```python
from build123d import *

# Parameters (mm, degrees)
SKETCH_1_W           = 40
SKETCH_1_H           = 15
EXTRUDE_1_DEPTH      = 5
CUT_EXTRUDE_START    = 5
SKETCH_2_R           = 5
SKETCH_2_R_2         = 1.5
CUT_EXTRUDE_1_DEPTH  = 5
EXTRUDE_3_DEPTH      = 8.75
EXTRUDE_3_DEPTH_BACK = 3.75
SKETCH_6_W           = 12.5
SKETCH_6_H           = 4
EXTRUDE_START        = 7.5
EXTRUDE_4_DEPTH      = 4
EXTRUDE_START_2      = -7.5
EXTRUDE_5_DEPTH      = 4
CUT_EXTRUDE_START_2  = 7.5
SKETCH_10_R          = 2.75
CUT_EXTRUDE_3_DEPTH  = 15
CUT_EXTRUDE_START_3  = -3.5
CUT_EXTRUDE_4_DEPTH  = 7
CHAMFER_1_SIZE       = 1


with BuildPart() as part:
    # 草图1 → 凸台-拉伸1 (new body)
    with BuildSketch(Plane(origin=(0, 0, 0), x_dir=(1, 0, 0), z_dir=(0, 1, 0))):
        Rectangle(SKETCH_1_W, SKETCH_1_H)
    extrude(amount=EXTRUDE_1_DEPTH)

    # 草图2 → 切除-拉伸1 (cut)
    with BuildSketch(Plane(origin=(0, 0, 0), x_dir=(1, 0, 0), z_dir=(0, 1, 0)).offset(CUT_EXTRUDE_START)):
        with Locations(Location((0, 0, 0), (0, 0, 90))):
            Circle(SKETCH_2_R)
        with Locations(Location((8, 0, 0), (0, 0, 90))):
            Circle(SKETCH_2_R_2)
        with Locations(Location((-8, 0, 0), (0, 0, 90))):
            Circle(SKETCH_2_R_2)
    extrude(amount=-CUT_EXTRUDE_1_DEPTH, mode=Mode.SUBTRACT)

    # 草图6 → 凸台-拉伸3 (add, two sides: drawn at the far end of the back side and taken through both)
    with BuildSketch(Plane(origin=(0, 0, 0), x_dir=(1, 0, 0), z_dir=(0, 1, 0)).offset(-EXTRUDE_3_DEPTH_BACK)):
        with Locations((26.25, 5.5)):
            Rectangle(SKETCH_6_W, SKETCH_6_H)
        with Locations((26.25, -5.5)):
            Rectangle(SKETCH_6_W, SKETCH_6_H)
        with Locations((-26.25, -5.5)):
            Rectangle(SKETCH_6_W, SKETCH_6_H)
        with Locations((-26.25, 5.5)):
            Rectangle(SKETCH_6_W, SKETCH_6_H)
    extrude(amount=EXTRUDE_3_DEPTH + EXTRUDE_3_DEPTH_BACK)

    # 草图8 → 凸台-拉伸4 (add)
    with BuildSketch(Plane.XY.offset(EXTRUDE_START)):
        Polygon((-20, -3.75), (-14, 0), (-20, 0), align=None)
        Polygon((-20, 8.75), (-14, 5), (-20, 5), align=None)
        Polygon((20, 0), (14, 0), (20, -3.75), align=None)
        Polygon((20, 5), (20, 8.75), (14, 5), align=None)
    extrude(amount=-EXTRUDE_4_DEPTH)

    # 草图9 → 凸台-拉伸5 (add)
    with BuildSketch(Plane.XY.offset(EXTRUDE_START_2)):
        Polygon((-14, 5), (-20, 8.75), (-20, 5), align=None)
        Polygon((-20, -3.75), (-14, 0), (-20, 0), align=None)
        Polygon((20, 5), (20, 8.75), (14, 5), align=None)
        Polygon((20, 0), (14, 0), (20, -3.75), align=None)
    extrude(amount=EXTRUDE_5_DEPTH)

    # 草图10 → 切除-拉伸3 (cut)
    with BuildSketch(Plane.XY.offset(CUT_EXTRUDE_START_2)):
        with BuildLine():
            Line((-32.5, 2.5), (-32.5, -3.75))
            Line((-32.5, -3.75), (-26.25, -3.75))
            ThreePointArc((-26.25, -3.75), (-30.669417382, -1.919417382), (-32.5, 2.5))
        make_face()
        with BuildLine():
            Line((-32.5, 8.75), (-32.5, 2.5))
            ThreePointArc((-32.5, 2.5), (-30.669417382, 6.919417382), (-26.25, 8.75))
            Line((-26.25, 8.75), (-32.5, 8.75))
        make_face()
        with Locations(Location((26.25, 2.5, 0), (0, 0, 180))):
            Circle(SKETCH_10_R)
        with BuildLine():
            ThreePointArc((32.5, 2.5), (30.669417382, -1.919417382), (26.25, -3.75))
            Line((26.25, -3.75), (32.5, -3.75))
            Line((32.5, -3.75), (32.5, 2.5))
        make_face()
        with BuildLine():
            ThreePointArc((26.25, 8.75), (30.669417382, 6.919417382), (32.5, 2.5))
            Line((32.5, 2.5), (32.5, 8.75))
            Line((32.5, 8.75), (26.25, 8.75))
        make_face()
        with Locations((-26.25, 2.5)):
            Circle(SKETCH_10_R)
    extrude(amount=-CUT_EXTRUDE_3_DEPTH, mode=Mode.SUBTRACT)

    # 草图11 → 切除-拉伸4 (cut)
    with BuildSketch(Plane.XY.offset(CUT_EXTRUDE_START_3)):
        with BuildLine():
            Line((20, 2.5), (20, 5))
            Line((20, 5), (17.5, 5))
            ThreePointArc((17.5, 5), (19.267766953, 4.267766953), (20, 2.5))
        make_face()
        with BuildLine():
            Line((20, 0), (20, 2.5))
            ThreePointArc((20, 2.5), (19.267766953, 0.732233047), (17.5, 0))
            Line((17.5, 0), (20, 0))
        make_face()
        with BuildLine():
            Line((-20, 0), (-17.5, 0))
            ThreePointArc((-17.5, 0), (-19.267766948, 0.732233042), (-20, 2.499999987))
            Line((-20, 2.499999987), (-20, 0))
        make_face()
        with BuildLine():
            Line((-20, 5), (-20, 2.499999987))
            ThreePointArc((-20, 2.499999987), (-19.267766958, 4.267766948), (-17.5, 5))
            Line((-17.5, 5), (-20, 5))
        make_face()
    extrude(amount=CUT_EXTRUDE_4_DEPTH, mode=Mode.SUBTRACT)

    # 倒角1
    chamfer_1_edges = [part.edges().sort_by_distance(p)[0] for p in [
        (17, -1.875, 7.5),
        (17, 6.875, 7.5),
        (-17, 6.875, -7.5),
        (-17, -1.875, -7.5),
        (0, 5, -7.5),
        (17, 6.875, -7.5),
        (0, 0, -7.5),
        (17, -1.875, -7.5),
        (-23.125, 8.75, 7.5),
        (23.125, -3.75, -7.5),
        (32.5, 2.5, 7.5),
        (32.5, 2.5, -7.5),
        (-32.5, 2.5, 7.5),
        (-32.5, 2.5, -7.5),
        (-23.125, -3.75, 7.5),
        (23.125, 8.75, -7.5),
        (23.125, -3.75, 7.5),
        (23.125, 8.75, 7.5),
        (-23.125, -3.75, -7.5),
        (-23.125, 8.75, -7.5),
        (0, 0, 7.5),
        (-17, -1.875, 7.5),
        (0, 5, 7.5),
        (-17, 6.875, 7.5),
    ]]
    chamfer(chamfer_1_edges, length=CHAMFER_1_SIZE)


solid = part.part
```
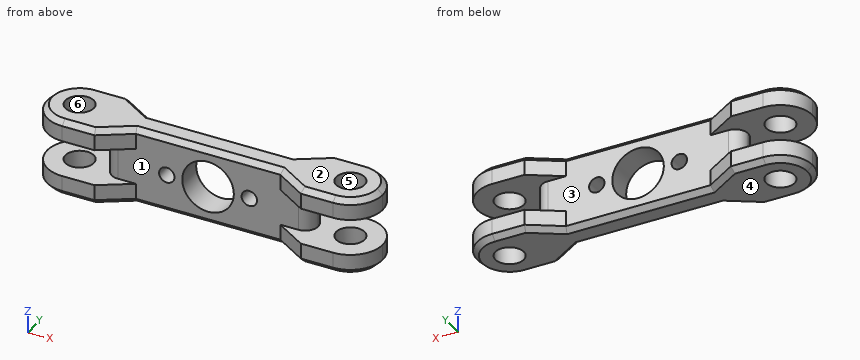
For this review, take the finished solid that the model builds, in its own axes (mm). Face numbers are marked on the shaded views. A direction names the side the tool comes from. Give positions to 0.01 mm unless a question says otherwise; leave off trailing zeros. Order: outer loops, then holes, each group sorted by start corner. A loop starts at its lowest first (then second) coordinate and runs counter-clockwise, first axis right, second up.
1) Take a section at B-B (z = 0). Give the boundary of the cut face in (x, y).
2) For the marked faces 1 and 2, list the 3-axis set-ups (+Z, -Z, +X, -X, +Y, -Y) from which the entire face can be reached by the end or side of a thin tool; tool diameter is ignored.
3) Insertion check: pin 1 (1 mm diameter, centred on x = -5, z = 2.5, fed in from -Y); pin 2 (3 mm diameter, centred on y = 3, z = 1, fed in from +X); pin 3 (1.5 mm diameter, centred on x = -6, z = 3, fed in from +Y). Each pin has a flat end and moves straight along its axis. Give the tip position at first contact, or say it passes through.
4) Wall thickness on line 1 (X direction, y = 2.7, z = 0); line 2 (Z direction, x = 8, y = 2.3); line 3 (X direction, y = 3.55, z = 0): over which ranges is each line inside the solid? List them lowest first.
5) Take a section at A-A (x = 0). Give the boundary of the cut face in (y, z).
6) Take a section at D-D (x = 8). Give the boundary of the cut face in (y, z), then the cut area to 3 significant figures.
7) Take a section at C-C (z = -4.25). Give the boundary of the cut face in (x, y), then the cut area to 3 significant figures.
8) The part is to be moulded in two halves that separate along Y. For the marked faces 3, 4, 5 and 6, say which applies: released by +Y, released by -Y, zero draft, split by the parting line, or undercut.
Derived:
1. outline: (-17.5, 0) - (-9.5, 0) - (-9.5, 5) - (-17.5, 5) arc R2.5 ccw to start; (-6.5, 0) - (-5, 0) - (-5, 5) - (-6.5, 5) - close; (5, 0) - (6.5, 0) - (6.5, 5) - (5, 5) - close; (9.5, 0) - (17.5, 0) arc R2.5 ccw to (17.5, 5) - (9.5, 5) - close
2. face 1: -Y
2. face 2: +Z, +X, -X, +Y, -Y
3. pin 1: stops at y = 0
3. pin 2: stops at x = 20
3. pin 3: stops at y = 5
4. line 1: x = -19.99 to -9.5, -6.5 to -5, 5 to 6.5, 9.5 to 19.99
4. line 2: z = -7.5 to -1.5, 1.5 to 7.5
4. line 3: x = -19.77 to -9.5, -6.5 to -5, 5 to 6.5, 9.5 to 19.77
5. outline: (0, -6.5) - (1, -7.5) - (4, -7.5) - (5, -6.5) - (5, -5) - (0, -5) - close; (0, 5) - (5, 5) - (5, 6.5) - (4, 7.5) - (1, 7.5) - (0, 6.5) - close
6. outline: (0, -6.5) - (1, -7.5) - (4, -7.5) - (5, -6.5) - (5, -1.5) - (0, -1.5) - close; (0, 1.5) - (5, 1.5) - (5, 6.5) - (4, 7.5) - (1, 7.5) - (0, 6.5) - close
6. area: 58.0 mm2
7. outline: (-26.25, -3.75) - (-20, -3.75) - (-14, 0) - (-2.63, 0) - (-2.63, 5) - (-14, 5) - (-20, 8.75) - (-26.25, 8.75) arc R6.25 ccw to start; (2.63, 0) - (14, 0) - (20, -3.75) - (26.25, -3.75) arc R6.25 ccw to (26.25, 8.75) - (20, 8.75) - (14, 5) - (2.63, 5) - close; hole circle Ø5.5 at (-26.25, 2.5); hole circle Ø5.5 at (26.25, 2.5)
7. area: 450 mm2
8. face 3: released by +Y
8. face 4: zero draft
8. face 5: undercut
8. face 6: undercut
